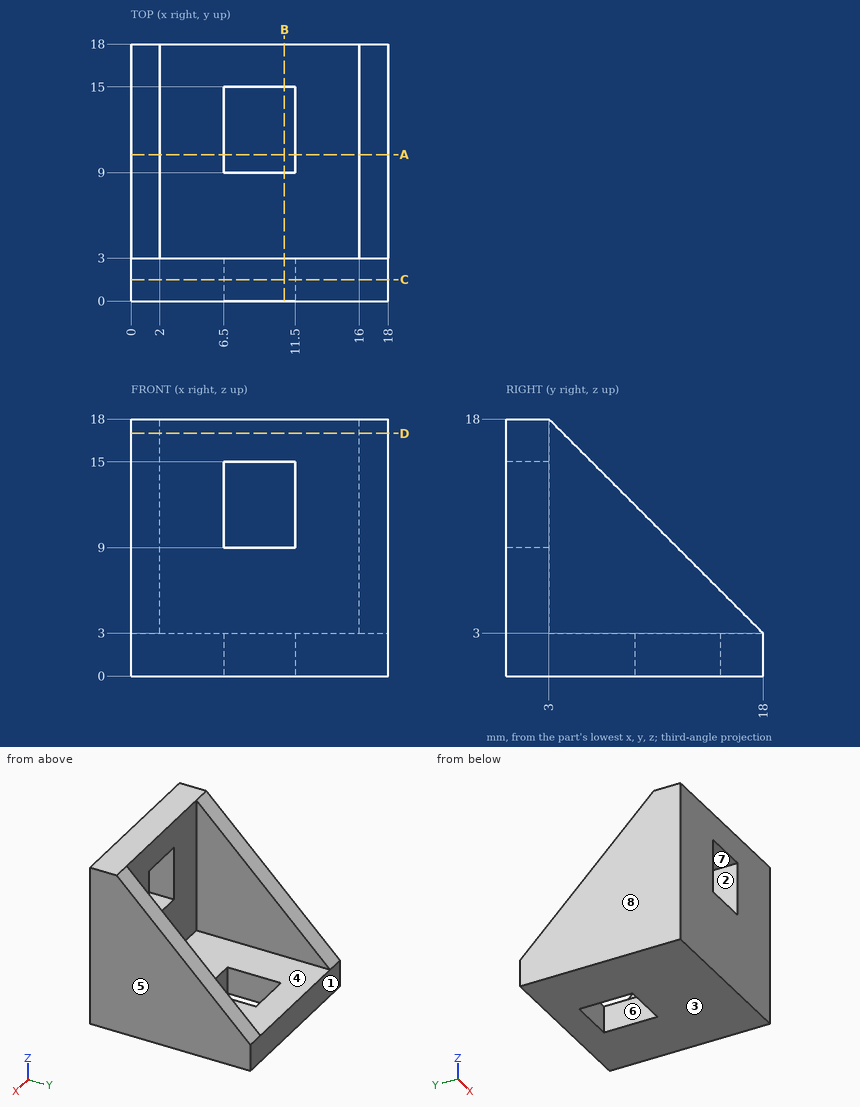
Geometry: see drawing. Coordinates: mm, zero at the bounding-box minimum. A direction names the side the tool comes from. Give positions to 0.01 mm unless a question says otherwise; leave off trailing zeros. Write each loop counter-clockwise with the first axis right and the second up, starting at its lowest first coordinate (ties: lowest second). Pieces come first, ordered by that corner, then holes. Notation, with made-up numbers: (57, 32) - (90, 32) arc R16 ccw to (90, 59) - close; hole circle Ø8 at (-20, 36.5). An arc over 180 degrees is marked (long way). Return JSON: item names as keys, results as strings. Group by question number.
1) Set-up query: the marked faces 4, 5, 6, 7 and 8. Return all of +Z, -Z, +X, -X, +Y, -Y with unobstructed straight access to the full face (end or side cutting, diameter ignored); none if empty.
2) First-contact query: P1, Ø1.5, axis at x = 8, z = 1.5, coming from the -Y side; P2, Ø4, axis at x = 8, y = 9.5, coming from the +Z side; P3, Ø1.5, axis at x = 2.5, z = 6.5, coming from the +Y side. Flat tips, straight axial feed; report the tip coordinate or a pass-through.
3) Mould query, pull axis Z, two halves, no side actions, for the marked faces 1, 2 and 3. Classes: released by +Z, released by -Z, zero draft, split by the parting line, or undercut.
4) Line query: line 1 (X direction, y = 7.5, z = 5.5); line 2 (Z direction, x = 13.5, y = 11). Output: solid intervals per line, ascending.
5) Section C-C on y = 1.5. Return the cut outline in (x, z).
6) Section B-B on x = 10.75. Return the cut outline in (y, z), plus the area to 3 significant figures.
7) Section D-D on z = 17. Return the cut outline in (x, y).
8) Section A-A on y = 10.25. Return the cut outline in (x, z), plus the area to 3 significant figures.
Filled in:
{
 "1": {"face 4": "+Z, +Y", "face 5": "+Z, -Z, +X, +Y, -Y", "face 6": "+Z, -Z", "face 7": "+Y, -Y", "face 8": "+Z, -Z, -X, +Y, -Y"},
 "2": {"P1": "stops at y = 0", "P2": "stops at z = 3", "P3": "stops at y = 15.06"},
 "3": {"face 1": "zero draft", "face 2": "undercut", "face 3": "released by -Z"},
 "4": {"line 1": "x = 0 to 2, 16 to 18", "line 2": "z = 0 to 3"},
 "5": {"outline": "(0, 0) - (18, 0) - (18, 18) - (0, 18) - close; hole (6.5, 9) - (11.5, 9) - (11.5, 15) - (6.5, 15) - close"},
 "6": {"outline": "(0, 0) - (9, 0) - (9, 3) - (3, 3) - (3, 9) - (0, 9) - close; (0, 15) - (3, 15) - (3, 18) - (0, 18) - close; (15, 0) - (18, 0) - (18, 3) - (15, 3) - close", "area": "63.0 mm^2"},
 "7": {"outline": "(0, 0) - (18, 0) - (18, 4) - (16, 4) - (16, 3) - (2, 3) - (2, 4) - (0, 4) - close"},
 "8": {"outline": "(0, 0) - (6.5, 0) - (6.5, 3) - (2, 3) - (2, 10.75) - (0, 10.75) - close; (11.5, 0) - (18, 0) - (18, 10.75) - (16, 10.75) - (16, 3) - (11.5, 3) - close", "area": "70.0 mm^2"}
}
